Verification items for the finished model (mm, model axes). A direction names the side the tool comes from. Round coordinates to 2 decimals unless told otherwise and drop trailing zeros. Answer as a JSON object with one key per item and string values.
Autodesk Inventor part; units mm, degrees
ref_plane "Work Plane1" through (27.5, 27.5, -160) normal (0, 0, -1) x (-1, 0, 0)
ref_plane "YZ Plane" through (0, 0, 0) normal (1, 0, 0) x (0, 1, 0)
ref_plane "XZ Plane" through (0, 0, 0) normal (0, 1, 0) x (-1, 0, 0)
sketch "Sketch1" plane through (0, 0, 0) normal (1, 0, 0) x (0, 1, 0)
  circle A0 centre (0, 0) radius 27.5
  line L0 (-27.5, 0) -> (-27.5, -60)
  line L1 (-27.5, -60) -> (27.5, -60)
  line L2 (27.5, -60) -> (27.5, 0)
  dimension "d0" = 55
  dimension "d1" = 60
extrude "Extrusion1" add sketch "Sketch1" along normal mid plane 55
sketch "Sketch2" plane through (27.5, 27.5, -60) normal (0, 0, -1) x (-1, 0, 0)
  line L0 (0, -55) -> (0, 0)
  line L1 (55, 0) -> (0, 0)
  line L2 (0, 0) -> (0, -55)
  line L3 (0, -55) -> (55, -55)
  line L4 (55, -55) -> (55, 0)
  line L5 (55, 0) -> (0, -55) construction
  line L6 (0, 0) -> (55, -55) construction
  point P0 (27.5, -27.5)
ref_plane "Work Plane1" through (27.5, 27.5, -160) normal (0, 0, -1) x (-1, 0, 0)
sketch "Sketch3" plane through (27.5, 27.5, -160) normal (0, 0, -1) x (-1, 0, 0)
  circle A0 centre (27.5, -27.5) radius 27.5
  line L0 (55, -55) -> (0, -55)
  point P0 (27.5, -27.5)
loft "Loft1" add profiles "Sketch2", "Sketch3"
sketch "Sketch4" plane through (27.5, 27.5, -160) normal (0, 0, -1) x (-1, 0, 0)
  circle A0 centre (27.5, -27.5) radius 15
  point P0 (27.5, -27.5)
  dimension "d9" = 30
extrude "Extrusion2" cut sketch "Sketch4" against normal blind 60
properties part number "shank"
Q1. Gauge pin test, flat ends, axial feed: P1, Ø1, axis at x = 7, z = 2, coming from the +Y side; P2, Ø1, axis at y = -13, z = -122, coming from the -X side; P3, Ø5, axis at x = -16, y = -4, coming from the +Z side. Record the tip position at first contact, or that the pin passes through.
Geometry check:
{"P1": "stops at y = 27.46", "P2": "stops at x = -26.03", "P3": "stops at z = 27.46"}
Q2. Release check for a two-part mould opening along X. For faces 1 (the flat face through (-27.5, 0, -16)), 2 (the flat face through (27.5, 0, -16)), 3 (the cylindrical face through (14.985, 0.66, -130.42)) record: released by +X, released by -X, zero draft, split by the parting line, or undercut.
Geometry check:
{"face 1": "released by -X", "face 2": "released by +X", "face 3": "undercut"}
Q3. Material ranges on line 1 along Y through (x, z) = (0, -126.5); line 2 along Z through (x, y) = (-8, 1); line 3 along Z through (x, y) = (15, -1), recorded low to high. Write a range as [from, to].
Geometry check:
{"line 1": "y = [-27.5, -15], [15, 27.5]", "line 2": "z = [-100, 27.48]", "line 3": "z = [-160, 27.48]"}
Q4. Set-up check for faces 4 (the flat face through (-12, -12, -160)), 5 (the flat face through (0, 0, -100)): record each of +Z, -Z, +X, -X, +Y, -Y from which the full face is reachable in a straight line by a thin tool's end or side.
Geometry check:
{"face 4": "-Z, +X, -X, +Y, -Y", "face 5": "-Z"}
